from build123d import *

# Parameters (mm, degrees)
SKETCH2_W                = 0.4
SKETCH2_H                = 16
SKETCH2_H_2              = 18
BOSS_EXTRUDE1_DEPTH      = 0.2
BOSS_EXTRUDE1_DEPTH_BACK = 0.2


with BuildPart() as part:
    # Sketch1 → Revolve1 (revolve)
    with BuildSketch(Plane.XY):
        with BuildLine():
            Line((0, 0), (2.7, 0))
            Line((2.7, 0), (2.7, 1))
            Line((2.7, 1), (2.5, 1))
            Line((2.5, 1), (2.5, 6.3))
            ThreePointArc((2.5, 6.3), (1.767766953, 8.067766953), (0, 8.8))
            Line((0, 8.8), (0, 0))
        make_face()
    revolve(axis=Axis((0, 8.8, 0), (0, -1, 0)))

    # Sketch2 → Boss-Extrude1 (add, two sides)
    with BuildSketch(Plane.XY) as boss_extrude1_sk:
        with Locations((1.35, -8)):
            Rectangle(SKETCH2_W, SKETCH2_H)
        with Locations((-1.35, -9)):
            Rectangle(SKETCH2_W, SKETCH2_H_2)
    extrude(amount=BOSS_EXTRUDE1_DEPTH)
    extrude(boss_extrude1_sk.sketch, amount=-BOSS_EXTRUDE1_DEPTH_BACK)


solid = part.part
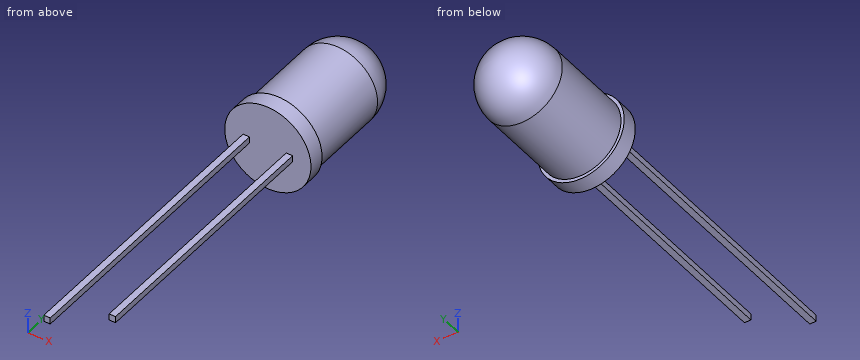
Could you check a few things on this model? Use its own coordinates, in mm. Coordinates: 2 decimals unless noted, no trailing zeros. Loops run counter-clockwise (first coordinate to the right, second up) from the corner with the lowest first, then second, coordinate; pieces in that order, holes last.
1. Imagine slicing it at A-A (y = -3.5). Please give me the cut outline in (x, z).
2. Imagine slicing it at C-C (z = 0.8). Please give me the cut outline in (x, y).
3. I need wall thicknesses on L1, parallel to X at y = -8.25, z = 0; L2, parallel to Y at x = -1.4, z = -0.4; L3, parallel to Z at x = 1.45, y = 1.5. Which ranges of each line are inside material? Lowest first, please.
4. For P1, Ø2, axis at x = -2, z = 1.5, coming from the +Y side; P2, Ø2.5, axis at x = 1.5, z = -1, coming from the +Y side; P3, Ø1, axis at y = -10, z = -0.5, coming from the +X side, each with a flat end and sliding along its axis, tell me the tip position at first contact or that it passes through.
5. Imagine slicing it at B-B (x = 0). Please give me the cut outline in (y, z), and give its area (3 significant figures).
Computed values:
1. outline: (-1.55, -0.2) - (-1.15, -0.2) - (-1.15, 0.2) - (-1.55, 0.2) - close; (1.15, -0.2) - (1.55, -0.2) - (1.55, 0.2) - (1.15, 0.2) - close
2. outline: (-2.58, 0) - (2.58, 0) - (2.58, 1) - (2.37, 1) - (2.37, 6.3) arc R2.37 ccw to (-2.37, 6.3) - (-2.37, 1) - (-2.58, 1) - close
3. L1: x = -1.55 to -1.15, 1.15 to 1.55
3. L2: y = 0 to 8.33
3. L3: z = -2.04 to 2.04
4. P1: stops at y = 8.3
4. P2: stops at y = 8.74
4. P3: stops at x = 1.55
5. outline: (0, -2.7) - (1, -2.7) - (1, -2.5) - (6.3, -2.5) arc R2.5 ccw to (6.3, 2.5) - (1, 2.5) - (1, 2.7) - (0, 2.7) - close
5. area: 41.7 mm2
